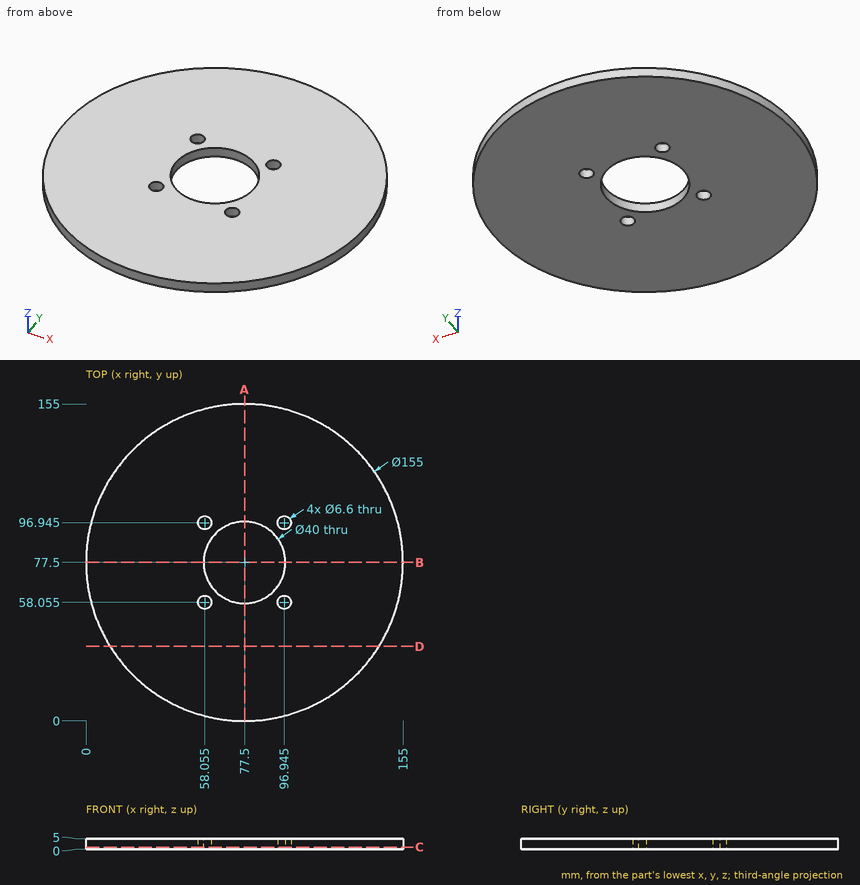
Can you work these out from the drawing? Everything is in mm from the part's minimum corner. Give positions to 0.01 mm unless a question says otherwise; leave off trailing zeros. Order: outer loops, then holes, each group sorted by start corner. A loop starts at its lowest first (then second) coordinate and runs counter-clockwise, first axis right, second up.
1. Suppose I cut it at D-D (y = 36.5). List the corners of the cut face in (x, z) for me.
2. Will these pins go through, and if not, where does the flat tip stop? P1, Ø1, axis at x = 66, z = 1.5, coming from the -Y side (1 decimal); P2, Ø1.5, axis at y = 28.5, z = 1.5, coming from the +X side.
3. I need wall thicknesses on L1, parallel to Y at x = 95.5, z = 2.75 (1 decimal); L2, parallel to Y at x = 77.5, z = 1.1; L3, parallel to Y at x = 61, z = 2.85 (1 decimal). Which ranges of each line are inside material? Lowest first, please.
4. Suppose I cut it at C-C (z = 1). List the corners of the cut face in (x, y) for me (1 decimal).
5. Suppose I cut it at A-A (x = 77.5). List the corners of the cut face in (y, z) for me.
Solved:
1. outline: (11.73, 0) - (143.27, 0) - (143.27, 5) - (11.73, 5) - close
2. P1: stops at y = 0.8
2. P2: stops at x = 138.15
3. L1: y = 2.1 to 55.1, 61 to 68.8, 86.2 to 94, 99.9 to 152.9
3. L2: y = 0 to 57.5, 97.5 to 155
3. L3: y = 1.8 to 56.6, 59.5 to 66.2, 88.8 to 95.5, 98.4 to 153.2
4. outline: circle Ø155 at (77.5, 77.5); hole circle Ø6.6 at (58.1, 58.1); hole circle Ø6.6 at (58.1, 96.9); hole circle Ø40 at (77.5, 77.5); hole circle Ø6.6 at (96.9, 58.1); hole circle Ø6.6 at (96.9, 96.9)
5. outline: (0, 0) - (57.5, 0) - (57.5, 5) - (0, 5) - close; (97.5, 0) - (155, 0) - (155, 5) - (97.5, 5) - close
